from build123d import *

# Parameters (mm, degrees)
SKETCH1_R           = 1.3
BOSS_EXTRUDE1_DEPTH = 5
SKETCH3_W           = 34
SKETCH3_H           = 17
SKETCH3_R           = 1.3
BOSS_EXTRUDE2_DEPTH = 4
FILLET1_R           = 3
FILLET2_R           = 3


with BuildPart() as part:
    # Sketch1 → Boss-Extrude1 (new body)
    with BuildSketch(Plane.XY):
        with BuildLine():
            Line((0, 50), (-17.67766953, 32.32233047))
            Line((-17.67766953, 32.32233047), (32.32233047, -17.67766953))
            Line((32.32233047, -17.67766953), (50, 0))
            ThreePointArc((50, 0), (35.355339059, 35.355339059), (0, 50))
        make_face()
        with Locations((47.7, 2.3)):
            Circle(SKETCH1_R, mode=Mode.SUBTRACT)
        with Locations((2.386492722, 47.695750885)):
            Circle(SKETCH1_R, mode=Mode.SUBTRACT)
        with Locations((7.050002215, 47.232165616)):
            Circle(SKETCH1_R, mode=Mode.SUBTRACT)
        with Locations((11.645616333, 46.313708772)):
            Circle(SKETCH1_R, mode=Mode.SUBTRACT)
        with Locations((16.129076799, 44.949225595)):
            Circle(SKETCH1_R, mode=Mode.SUBTRACT)
        with Locations((20.457205439, 43.151856804)):
            Circle(SKETCH1_R, mode=Mode.SUBTRACT)
        with Locations((24.588320007, 40.938912043)):
            Circle(SKETCH1_R, mode=Mode.SUBTRACT)
        with Locations((28.482635612, 38.331703179)):
            Circle(SKETCH1_R, mode=Mode.SUBTRACT)
        with Locations((32.102647866, 35.355339059)):
            Circle(SKETCH1_R, mode=Mode.SUBTRACT)
        with Locations((35.413494072, 32.038483697)):
            Circle(SKETCH1_R, mode=Mode.SUBTRACT)
        with Locations((38.383288971, 28.413080223)):
            Circle(SKETCH1_R, mode=Mode.SUBTRACT)
        with Locations((40.983431815, 24.514043255)):
            Circle(SKETCH1_R, mode=Mode.SUBTRACT)
        with Locations((43.188881806, 20.378922649)):
            Circle(SKETCH1_R, mode=Mode.SUBTRACT)
        with Locations((44.978399257, 16.047541877)):
            Circle(SKETCH1_R, mode=Mode.SUBTRACT)
        with Locations((46.334750135, 11.561614505)):
            Circle(SKETCH1_R, mode=Mode.SUBTRACT)
        with Locations((47.24487204, 6.964342465)):
            Circle(SKETCH1_R, mode=Mode.SUBTRACT)
    boss_extrude1 = extrude(amount=BOSS_EXTRUDE1_DEPTH)

    # Sketch3 → Boss-Extrude2 (add)
    with BuildSketch(Plane(origin=(7.32233047, 7.32233047, 0), x_dir=(-0.7071067811865535, 0.7071067811865417, 0), z_dir=(-0.7071067811865417, -0.7071067811865535, 0))):
        with Locations((0, -4)):
            Rectangle(SKETCH3_W, SKETCH3_H)
        with Locations(Location((0, 2, 0), (0, 0, 180))):
            Circle(SKETCH3_R, mode=Mode.SUBTRACT)
        with Locations(Location((14.5, 2, 0), (0, 0, 180))):
            Circle(SKETCH3_R, mode=Mode.SUBTRACT)
        with Locations((-14.5, 2)):
            Circle(SKETCH3_R, mode=Mode.SUBTRACT)
    boss_extrude2 = extrude(amount=BOSS_EXTRUDE2_DEPTH)

    # Mirror1: Boss-Extrude2 across plane
    add(boss_extrude2.mirror(Plane.XY.offset(12.5)))

    # Mirror2: Boss-Extrude1 across plane
    add(boss_extrude1.mirror(Plane.XY.offset(12.5)))

    # Fillet1
    fillet1_edges = [part.edges().sort_by_distance(p)[0] for p in [
        (19.343145751, -4.69848481, 22.5),
    ]]
    fillet(fillet1_edges, radius=FILLET1_R)

    # Fillet2
    fillet2_edges = [part.edges().sort_by_distance(p)[0] for p in [
        (-4.69848481, 19.343145751, 22.5),
        (-4.69848481, 19.343145751, 2.5),
        (19.343145751, -4.69848481, 2.5),
    ]]
    fillet(fillet2_edges, radius=FILLET2_R)


solid = part.part
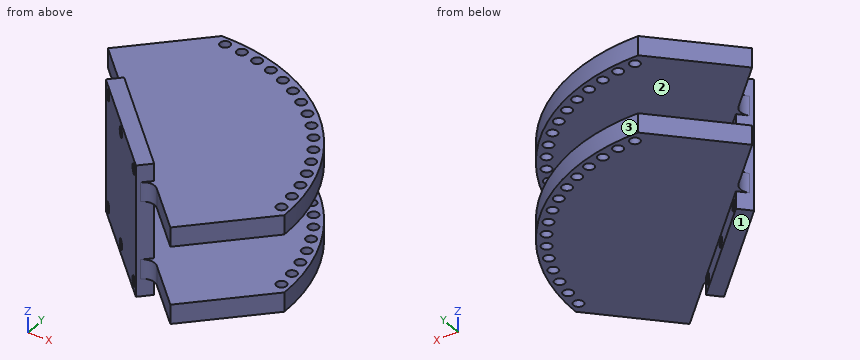
The model under review builds one solid part; all positions refer to its coordinate system, in mm. Face numbers are marked on the shaded views. Give positions to 0.01 mm unless a question says otherwise; leave off trailing zeros. Loops run counter-clockwise (first coordinate to the right, second up) from the corner with the lowest first, then second, coordinate; pieces in that order, holes last. Notation, with made-up numbers: (5.25, 1.25) -> (11.25, 1.25) arc R26 ccw to (11.25, 39.25) -> close; hole circle Ø2 at (12.5, 64). An arc over 180 degrees is marked (long way). Put each result on its own line as item: value. Start each with the question number.
1. We need section B-B on y = 2.3. State the section outline as (x, z) points.
2. We need section C-C on x = -12. State the section outline as (y, z) points.
3. We need section A-A on y = -10.5. State the section outline as (x, z) points.
4. Clearance check with flat-ended pins moving along their axes: P1, Ø3, axis at x = 24.59, y = 40.94, coming from the +Z side; P2, Ø2, axis at x = 17, y = 15, coming from the -Z side; P3, Ø2.5, axis at x = 20.46, y = 43.15, coming from the +Z side; P4, Ø10, axis at y = 20, z = 7, coming from the +X side. State where each tip first meets the part, or that it passes through.
5. We need section D-D on z = 8. State the section outline as (x, y) points.
6. Wall thickness on probe 1 along Z at (x, y) = (33.5, 1); probe 2 along Y at (x, z) = (45.5, 1); probe 3 along X at (y, z) = (19.5, 4): over which ranges is each line inside the solid? List them lowest first.
7. Mouldability with a two-part tool opening along Z and no side actions: class the marked faces 1, 2 and 3 as released by +Z, released by -Z, zero draft, split by the parting line, or undercut.
Determined:
1. outline: (6.69, -4.5) -> (12.34, -4.5) -> (12.34, 0) -> (46.4, 0) -> (46.4, 5) -> (12.34, 5) -> (12.34, 20) -> (46.4, 20) -> (46.4, 25) -> (12.34, 25) -> (12.34, 29.5) -> (6.69, 29.5) -> close; (49, 0) -> (49.95, 0) -> (49.95, 5) -> (49, 5) -> close; (49, 20) -> (49.95, 20) -> (49.95, 25) -> (49, 25) -> close
2. outline: (26.64, 0) -> (38, 0) -> (38, 5) -> (26.64, 5) -> close; (26.64, 20) -> (38, 20) -> (38, 25) -> (26.64, 25) -> close
3. outline: (25.14, 0) -> (39.5, 0) -> (39.5, 5) -> (25.14, 5) -> close; (25.14, 20) -> (39.5, 20) -> (39.5, 25) -> (25.14, 25) -> close
4. P1: z = 25
4. P2: z = 0
4. P3: through
4. P4: x = 47.56
5. outline: (-7.53, 16.51) -> (16.51, -7.53) -> (19.34, -4.7) -> (-4.7, 19.34) -> close
6. probe 1: 0 to 5, 20 to 25
6. probe 2: -4.5 to 10.57, 12.56 to 14.86, 17.24 to 20.73
6. probe 3: -5.95 to 42.23, 44.15 to 46.04
7. face 1: released by -Z
7. face 2: undercut
7. face 3: zero draft
